The figure shows three views and two pictorial views of one solid part (mm, origin at its lowest corner). Answer the questions. A direction names the side the tool comes from. Round coordinates to 2 decimals unless told otherwise and drop trailing zeros. Order: outer loops, then holes, each group sorted by start corner. A loop starts at its lowest first (then second) coordinate and runs counter-clockwise, first axis right, second up. Notation, with made-up numbers: (-37, -29.75) - (-25, -29.75) arc R21 cw to (-25, 8.25) - close; hole circle Ø6 at (17, 73.5). An arc over 180 degrees is marked (long way). Answer in a Markdown table with one row per item.
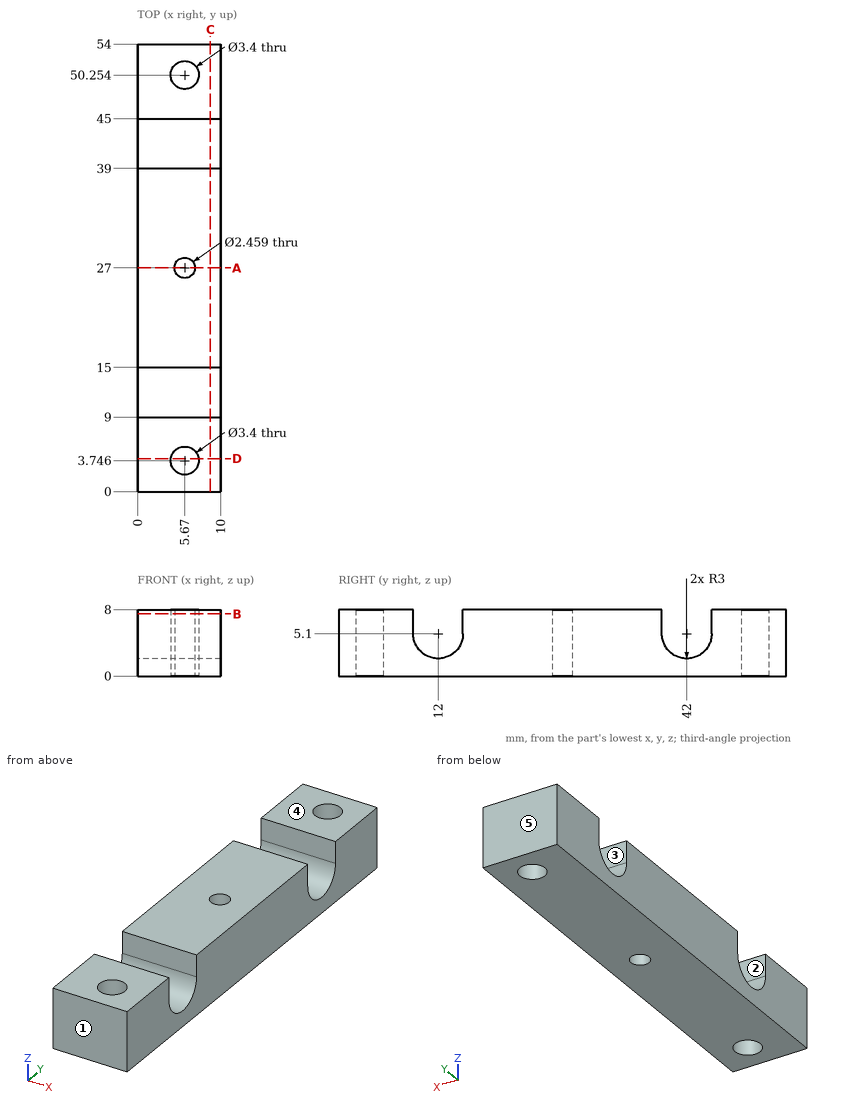
1) Find section C-C, the plane x = 8.75. Give the vertices of the cut face in (y, z), then the cut area to 3 significant figures.
Filled in:
| item | result |
|---|---|
| outline | (0, 0) - (54, 0) - (54, 8) - (45, 8) - (45, 5.1) arc R3 cw to (39, 5.1) - (39, 8) - (15, 8) - (15, 5.1) arc R3 cw to (9, 5.1) - (9, 8) - (0, 8) - close |
| area | 369 mm^2 |
2) Find section B-B, the plane z = 7.5. Give the vertices of the cut face in (x, y).
Filled in:
| item | result |
|---|---|
| outline | (0, 0) - (10, 0) - (10, 9) - (0, 9) - close; (0, 15) - (10, 15) - (10, 39) - (0, 39) - close; (0, 45) - (10, 45) - (10, 54) - (0, 54) - close; hole circle Ø3.4 at (5.67, 3.75); hole circle Ø3.4 at (5.67, 50.25); hole circle Ø2.46 at (5.67, 27) |
3) This flat-tipped pin is pushed along its axis until it touches: pin 1 (2 mm diameter, centred on x = 5.67, y = 3.75, fed in from +Z). Where does it stop, or does it pass through?
Filled in:
| item | result |
|---|---|
| pin 1 | passes through |
4) Find section D-D, the plane y = 4. Give the vertices of the cut face in (x, z), then the cut area to 3 significant figures.
Filled in:
| item | result |
|---|---|
| outline | (0, 0) - (3.99, 0) - (3.99, 8) - (0, 8) - close; (7.35, 0) - (10, 0) - (10, 8) - (7.35, 8) - close |
| area | 53.1 mm^2 |
5) Find section A-A, the plane y = 27. Give the vertices of the cut face in (x, z).
Filled in:
| item | result |
|---|---|
| outline | (0, 0) - (4.44, 0) - (4.44, 8) - (0, 8) - close; (6.9, 0) - (10, 0) - (10, 8) - (6.9, 8) - close |
6) The mould has two halves that part along Y. Classify the marked faces 3, 4 and 5: released by +Y, released by -Y, zero draft, split by the parting line, or undercut.
Filled in:
| item | result |
|---|---|
| face 3 | undercut |
| face 4 | zero draft |
| face 5 | released by +Y |
7) Which of the six approach directions +Z, -Z, +X, -X, +Y, -Y give full straight-line access (tool end or side, diameter ignored) to the marked faces 1 and 2?
Filled in:
| item | result |
|---|---|
| face 1 | +Z, -Z, +X, -X, -Y |
| face 2 | +Z, +X, -X |
8) Find the intervals of material crossed by probe 1 along Y at (x, z) = (3, 7.5); probe 2 along Y at (x, z) = (5.5, 7.5) (1 decimal); probe 3 along X at (y, z) = (27, 3), in increasing order. Write a range as from..to.
Filled in:
| item | result |
|---|---|
| probe 1 | y = 0..9, 15..39, 45..54 |
| probe 2 | y = 0..2.1, 5.4..9, 15..25.8, 28.2..39, 45..48.6, 51.9..54 |
| probe 3 | x = 0..4.44, 6.9..10 |
